The listing builds one solid part. Answer for the finished solid, in the listing's coordinates (mm). A direction names the side the tool comes from. Round coordinates to 2 decimals unless told otherwise and drop trailing zeros. Order: outer loops, then holes, each group sorted by start corner. A loop starts at its lowest first (then second) coordinate and runs counter-clockwise, first axis right, second up. Notation, with made-up numbers: M 88.25,-9 L 125.25,-9 A14 cw 125.25,17 Z; hole C -1,61.25 d2. An arc over 180 degrees is marked long. Write item = value, one per line. Start each with the question number.
(1) A cutting plane is placed at A-A, the plane x = -7.5. Determine the outline of the cut face in (y, z), and give its area (3 significant figures).
(2) A cutting plane is placed at C-C, the plane y = -204. Determine the outline of the cut face in (x, z).
(3) For a pull along Z with two mould halves and no side action, classify faces 1 (the face through (-5.555, -142.97, 2.526)), 2 (the face through (-14.8, 0, 7.5)), 3 (the face through (-10.7, -10.1, 4.6)) as released by +Z, released by -Z, zero draft, split by the parting line, or undercut.
(4) Which of the six approach directions +Z, -Z, +X, -X, +Y, -Y give full straight-line access (tool end or side, diameter ignored) to faces 4 (the face through (-14.8, -290, 7.5)), 5 (the face through (-14.078, -279.86, 3.412))?
(5) Each of these flat-tipped pins is pushed along its axis until it touches: pin 1 (3 mm diameter, centred on x = -12.95, z = 5.59, fed in from +Y); pin 2 (4 mm diameter, centred on x = -12.95, z = 5.59, fed in from -Y); pin 3 (5 mm diameter, centred on x = -9, y = -184.5, fed in from -Z). Where does it stop, or does it pass through?
(6) A cutting plane is placed at B-B, the plane z = 0.75. Determine the outline of the cut face in (x, y).
(7) Straight lines are drawn through the part: probe 1 along Z at (x, y) = (-12.5, -189); probe 2 along X at (y, z) = (-188, 5.5); probe 3 along X at (y, z) = (-270.5, 6.25). For each, find the intervals that lie inside material, in ascending order. Write a range as from..to.
from build123d import *

# Parameters (mm, degrees)
F0_R     = 8
F1_DEPTH = 290
F3_D     = 4.91
F3_DEPTH = 20
F3_TIP   = 1.4751128197
F5_D     = 4.91
F5_DEPTH = 20
F5_TIP   = 1.4751128197


with BuildPart() as f1:
    # F0 (on Front) → F1 (new body)
    with BuildSketch(Plane.XZ):
        with Locations((-12.9452068359, 5.5899755098)):
            Circle(F0_R)
    extrude(amount=F1_DEPTH)

    # F3
    with Locations(Plane.XZ.offset(290)):
        with Locations((-12.9452068359, 5.5899755098)):
            Hole(F3_D / 2, depth=F3_DEPTH)
            with Locations((0, 0, -(F3_DEPTH + F3_TIP / 2))):  # 118° drill point
                Cone(0, F3_D / 2, F3_TIP, mode=Mode.SUBTRACT)

    # F5
    with Locations(Plane(origin=(0, 0, 0), x_dir=(-1, 0, 0), z_dir=(0, 1, 0))):
        with Locations((12.9452068359, 5.5899755098)):
            Hole(F5_D / 2, depth=F5_DEPTH)
            with Locations((0, 0, -(F5_DEPTH + F5_TIP / 2))):  # 118° drill point
                Cone(0, F5_D / 2, F5_TIP, mode=Mode.SUBTRACT)


solid = f1.part
Reported:
q1.outline = M -290,-0.27 L 0,-0.27 L 0,11.45 L -290,11.45 Z
q1.area = 3,400 mm²
q2.outline = C -12.95,5.59 d16
q3.face_1 = split by the parting line
q3.face_2 = zero draft
q3.face_3 = undercut
q4.face_4 = +Z, -Z, +X, -X, -Y
q4.face_5 = -Y
q5.pin_1 = -20.57
q5.pin_2 = -269.73
q5.pin_3 = -2.28
q6.outline = M -19.32,-290 L -6.58,-290 L -6.58,0 L -19.32,0 Z
q7.probe_1 = -2.4..13.58
q7.probe_2 = -20.94..-4.95
q7.probe_3 = -20.92..-15.31, -10.58..-4.97
